from build123d import *

# Parameters (mm, degrees)
F1_DEPTH    = 6
F2_F1_R     = 0.2
F2_F2_R     = 0.2
F3_T4_DEPTH = 28.4585903453
F3_T9_DEPTH = 28.4585903453
F4_R        = 5.99999


# Not quite as in the source:
# - a fillet or chamfer that OpenCascade refuses, or shapes differently, is made with other operations: its cross-section is extruded or revolved along the edge and cut away or added
# - a fillet or chamfer is up to 0.001 mm smaller than in the source, because OpenCascade refuses the exact size


with BuildPart() as f1:
    # F0 (on Top) → F1 (new body)
    with BuildSketch(Plane.XY):
        Polygon((-7.5, 8), (-4.418584287, -3.5), (4.418584287, -3.5), (7.5, 8), align=None)
        with BuildLine():
            ThreePointArc((-1.5, 1.5), (-2.5606601718, 4.0606601718), (0, 3))
            ThreePointArc((0, 3), (2.5606601718, 4.0606601718), (1.5, 1.5))
            ThreePointArc((1.5, 1.5), (2.5606601718, -1.0606601718), (0, 0))
            ThreePointArc((0, 0), (-2.5606601718, -1.0606601718), (-1.5, 1.5))
        make_face(mode=Mode.SUBTRACT)
        Polygon((-9, -5), (-9, -7), (9, -7), (9, -5), (4.0166604984, -5), (-4.0166604984, -5), align=None)
        Polygon((-4.418584287, -3.5), (-4.0166604984, -5), (4.0166604984, -5), (4.418584287, -3.5), align=None)
    extrude(amount=F1_DEPTH)

    # F2: fillet of radius 0.2 on 4 edges, made by hand

    # F2_f1
    f2_f1_edges = [f1.edges().sort_by_distance(p)[0] for p in [
        (-1.5, 1.5, 3),
        (0, 3, 3),
        (1.5, 1.5, 3),
    ]]
    fillet(f2_f1_edges, radius=F2_F1_R)

    # F2_f2
    f2_f2_edges = [f1.edges().sort_by_distance(p)[0] for p in [
        (0, 0, 3),
    ]]
    fillet(f2_f2_edges, radius=F2_F2_R)

    # F3: fillet of radius 3 on 2 edges, made by hand


with BuildPart() as f3_tool2:
    # F3_s3 → F3_t4 (new body)
    with BuildSketch(Plane(origin=(-4.4435475741, 16.5835453123, 0), x_dir=(0, 0, 1), z_dir=(0.2588190451, -0.9659258263, 0))):
        with BuildLine():
            ThreePointArc((3, 5.1738913363), (5.1213203436, 4.2952116799), (6, 2.1738913363))
            Line((6, 2.1738913363), (6, 5.1738913363))
            Line((6, 5.1738913363), (3, 5.1738913363))
        make_face()
    extrude(amount=F3_T4_DEPTH)

    split(bisect_by=Plane.XZ.offset(5), keep=Keep.BOTTOM)


with BuildPart() as f1_1:
    add(f1.part)

    # F3_t1: cut F3_tool2
    add(f3_tool2.part, mode=Mode.SUBTRACT)


with BuildPart() as f3_tool7:
    # F3_s8 → F3_t9 (new body)
    with BuildSketch(Plane(origin=(-2.9220776041, -10.905342082, 0), x_dir=(0, 0, 1), z_dir=(0.2588190451, 0.9659258263, 0))):
        with BuildLine():
            ThreePointArc((3, 5.1738913363), (5.1213203436, 4.2952116799), (6, 2.1738913363))
            Line((6, 2.1738913363), (6, 5.1738913363))
            Line((6, 5.1738913363), (3, 5.1738913363))
        make_face()
    extrude(amount=F3_T9_DEPTH)

    split(bisect_by=Plane.XZ.offset(5), keep=Keep.BOTTOM)


with BuildPart() as f1_2:
    add(f1_1.part)

    # F3_t6: cut F3_tool7
    add(f3_tool7.part, mode=Mode.SUBTRACT)

    # F4 (radius 6 in the source; OpenCascade refuses exactly that, so slightly less here)
    f4_edges = [f1_2.edges().sort_by_distance(p)[0] for p in [
        (9, -6, 6),
        (-9, -6, 6),
    ]]
    fillet(f4_edges, radius=F4_R)


solid = f1_2.part
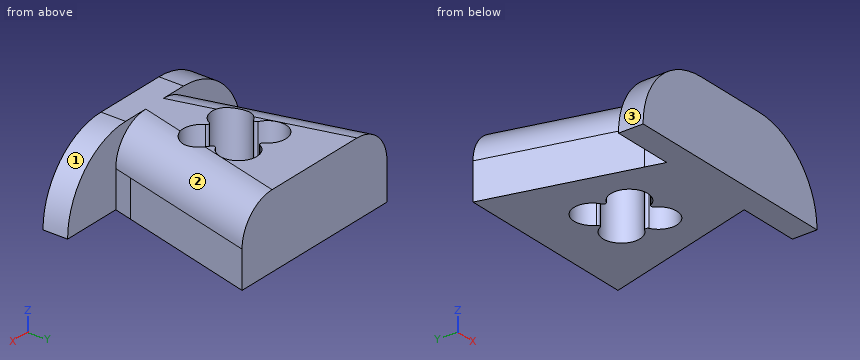
Geometry check sheet. Reference: the model listing, model coordinates, mm. Face numbers are marked on the shaded views. A direction names the side the tool comes from. Round coordinates to 2 decimals unless told otherwise and drop trailing zeros. Answer as a JSON object with one key per item and string values. Group by question number.
Item 1: Set-up check for the marked faces 1, 2 and 3: record each of +Z, -Z, +X, -X, +Y, -Y from which the full face is reachable in a straight line by a thin tool's end or side.
Item 2: Depth check by flat-ended pin: pin 1 Ø2.5 at (x, y) = (1.5, 0) entering from +Z; pin 2 Ø1.5 at (x, y) = (4, 2) entering from -Z; pin 3 Ø5 at (x, y) = (-6, -0.5) entering from +Z; pin 4 Ø1.5 at (y, z) = (3.5, 2.5) entering from -X. Enter the tip coordinate at first touch or a pass-through.
Item 3: Thickness scan on line 1 along Y through (x, z) = (-1.5, 1.75); line 2 along X through (y, z) = (1.5, 5); line 3 along X through (y, z) = (3, 3). Record the ranges inside material, lowest first.
Determined:
{
 "1": {"face 1": "+Z, +X, -Y", "face 2": "+Z, +X", "face 3": "+Z, -X, -Y"},
 "2": {"pin 1": "passes through", "pin 2": "stops at z = 0", "pin 3": "stops at z = 5.73", "pin 4": "stops at x = -6.5"},
 "3": {"line 1": "y = -7 to -1.5, 4.5 to 8", "line 2": "x = -4.97 to -2.1, 2.1 to 4.97", "line 3": "x = -6.16 to -3, 3 to 6.16"}
}
